```python
from build123d import *

# Parameters (mm, degrees)
BOSS_EXTRUDE1_DEPTH = 400
SKETCH2_R           = 7
CUT_EXTRUDE1_DEPTH  = 10


with BuildPart() as part:
    # Sketch1 → Boss-Extrude1 (new body)
    with BuildSketch(Plane(origin=(0, 0, 0), x_dir=(1, 0, 0), z_dir=(0, 1, 0))):
        with BuildLine():
            Line((-27.499872145, 29.213153277), (-67.499872145, 29.213153277))
            Line((-67.499872145, 29.213153277), (-67.499872145, -10.786846723))
            Line((-67.499872145, -10.786846723), (-66.499872145, -10.786846723))
            ThreePointArc((-66.499872145, -10.786846723), (-64.378551801, -9.908167067), (-63.499872145, -7.786846723))
            Line((-63.499872145, -7.786846723), (-63.499872145, 22.213153277))
            ThreePointArc((-63.499872145, 22.213153277), (-62.621192489, 24.334473621), (-60.499872145, 25.213153277))
            Line((-60.499872145, 25.213153277), (-30.499872145, 25.213153277))
            ThreePointArc((-30.499872145, 25.213153277), (-28.378551801, 26.091832933), (-27.499872145, 28.213153277))
            Line((-27.499872145, 28.213153277), (-27.499872145, 29.213153277))
        make_face()
    extrude(amount=BOSS_EXTRUDE1_DEPTH)

    # Sketch2 → Cut-Extrude1 (cut)
    with BuildSketch(Plane(origin=(-63.499872145, 0, 0), x_dir=(0, 0, -1), z_dir=(1, 0, 0))):
        with Locations((9.213153277, 200)):
            Circle(SKETCH2_R)
        with Locations((9.213153277, 50)):
            Circle(SKETCH2_R)
        with Locations((9.213153277, 350)):
            Circle(SKETCH2_R)
    extrude(amount=-CUT_EXTRUDE1_DEPTH, mode=Mode.SUBTRACT)


solid = part.part
```
Design review of the part built by this model. Coordinates are the model's own, in mm. A direction names the side the tool comes from. Give positions to 0.01 mm unless a question says otherwise; leave off trailing zeros. Loops run counter-clockwise (first coordinate to the right, second up) from the corner with the lowest first, then second, coordinate; pieces in that order, holes last. Notation, with made-up numbers: M -15.75,-33 L 8.25,-33 A21 ccw 8.25,-17 Z; hole C -3.5,6 d11. An arc over 180 degrees is marked long. Return JSON: item names as keys, results as strings. Group by question number.
Item 1: We need section C-C (y = 200). Give the boundary of the cut face in (x, z).
Item 2: For probe 1 along Z at (x, y) = (-66.2, 350); probe 2 along Z at (x, y) = (-48, 317); probe 3 along X at (y, z) = (152, -1), list the stretches that pass through material, from the lowest coordinate up.
Item 3: Tool access review of faces 1 (the flat face through (-63.5, 197, 0)), 2 (the flat face through (-67.5, 197, -18)): name each direction out of +Z, -Z, +X, -X, +Y, -Y from which nothing blocks a thin tool from reaching the whole face with its end or side.
Item 4: Insertion check: pin 1 Ø22.5 at (y, z) = (200, -9.21) entering from +X; pin 2 Ø12 at (x, y) = (-57, 149) entering from +Z; pin 3 Ø12.5 at (y, z) = (50, -9.21) entering from -X; pin 4 Ø24 at (x, y) = (-42.5, 104) entering from +Z. Each pin has a flat end and moves straight along its axis. Give the tip position at first contact, or say it passes through.
Item 5: Mouldability with a two-part tool opening along Z and no side actions: class faces 3 (the cylindrical face through (-65.472, 343.166, -7.696)), 4 (the flat face through (-46, 197, -25.213)), 5 (the flat face through (-47, 197, -29.213)) as released by +Z, released by -Z, zero draft, split by the parting line, or undercut.
Item 6: We need section A-A (y = 251). Give the boundary of the cut face in (x, z), and give its area (3 significant figures).
Item 7: We need section D-D (x = -36). Give the boundary of the cut face in (y, z), and give its area (3 significant figures).
Item 8: We need section B-B (z = -12.5). Give the boundary of the cut face in (x, y).
Output:
{
 "1": {"outline": "M -67.5,-29.21 L -27.5,-29.21 L -27.5,-28.21 A3 ccw -30.5,-25.21 L -60.5,-25.21 A3 cw -63.5,-22.21 L -63.5,-16.21 L -67.5,-16.21 Z; M -67.5,-2.21 L -63.5,-2.21 L -63.5,7.79 A3 ccw -66.5,10.79 L -67.5,10.79 Z"},
 "2": {"probe 1": "z = -29.21 to -16.21, -2.21 to 10.77", "probe 2": "z = -29.21 to -25.21", "probe 3": "x = -67.5 to -63.5"},
 "3": {"face 1": "+Z, +X, +Y, -Y", "face 2": "+Z, -Z, -X, +Y, -Y"},
 "4": {"pin 1": "stops at x = -63.5", "pin 2": "stops at z = -23.87", "pin 3": "passes through", "pin 4": "stops at z = -25.21"},
 "5": {"face 3": "undercut", "face 4": "released by +Z", "face 5": "released by -Z"},
 "6": {"outline": "M -67.5,-29.21 L -27.5,-29.21 L -27.5,-28.21 A3 ccw -30.5,-25.21 L -60.5,-25.21 A3 cw -63.5,-22.21 L -63.5,7.79 A3 ccw -66.5,10.79 L -67.5,10.79 Z", "area": "302 mm^2"},
 "7": {"outline": "M 0,-29.21 L 400,-29.21 L 400,-25.21 L 0,-25.21 Z", "area": "1,600 mm^2"},
 "8": {"outline": "M -67.5,0 L -63.5,0 L -63.5,43.82 L -67.5,43.82 Z; M -67.5,56.18 L -63.5,56.18 L -63.5,193.82 L -67.5,193.82 Z; M -67.5,206.18 L -63.5,206.18 L -63.5,343.82 L -67.5,343.82 Z; M -67.5,356.18 L -63.5,356.18 L -63.5,400 L -67.5,400 Z"}
}
